Work out the finished part from the listing and answer in its coordinate system (mm). Face numbers are marked on the shaded views. A direction names the side the tool comes from. Round coordinates to 2 decimals unless told otherwise and drop trailing zeros. Write each loop counter-clockwise with the first axis right and the second up, starting at its lowest first coordinate (ties: lowest second). Pieces come first, ordered by that corner, then holes. Notation, with made-up numbers: (-15, -0.5) - (-4, -0.5) arc R26 cw to (-4, 22.5) - close; hole circle Ø7 at (-26.5, 66). An arc over 180 degrees is marked (long way). Write item = value, one per line. Start each with the question number.
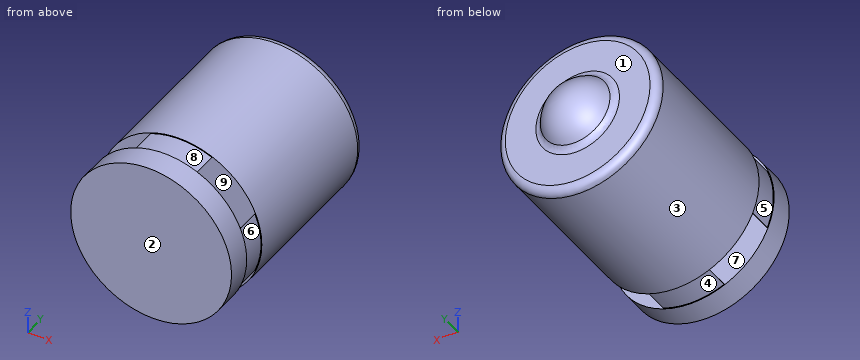
from build123d import *

# Parameters (mm, degrees)
SKETCH1_R           = 100
BOSS_EXTRUDE1_DEPTH = 30
BOSS_EXTRUDE2_DEPTH = 30
SKETCH3_R           = 100
BOSS_EXTRUDE3_DEPTH = 200
FILLET1_R           = 10
SCALE1_SCALE        = 0.233333333


with BuildPart() as part:
    # Sketch1 → Boss-Extrude1 (new body)
    with BuildSketch(Plane(origin=(0, 0, 0), x_dir=(1, 0, 0), z_dir=(0, 1, 0))):
        Circle(SKETCH1_R)
    extrude(amount=BOSS_EXTRUDE1_DEPTH)

    # Sketch2 → Boss-Extrude2 (add)
    with BuildSketch(Plane(origin=(0, 30, 0), x_dir=(1, 0, 0), z_dir=(0, 1, 0))):
        with BuildLine():
            Line((91.464073719, 37.885659804), (91.002133952, 37.694318088))
            ThreePointArc((91.002133952, 37.694318088), (98.5, 0), (91.002133952, -37.694318088))
            Line((91.002133952, -37.694318088), (91.464073719, -37.885659804))
            ThreePointArc((91.464073719, -37.885659804), (99, 0), (91.464073719, 37.885659804))
        make_face()
        with BuildLine():
            Line((37.885659804, -91.464073719), (37.694318088, -91.002133952))
            ThreePointArc((37.694318088, -91.002133952), (0, -98.5), (-37.694318088, -91.002133952))
            Line((-37.694318088, -91.002133952), (-37.885659804, -91.464073719))
            ThreePointArc((-37.885659804, -91.464073719), (0, -99), (37.885659804, -91.464073719))
        make_face()
        with BuildLine():
            Line((-91.464073719, -37.885659804), (-91.002133952, -37.694318088))
            ThreePointArc((-91.002133952, -37.694318088), (-98.5, 0), (-91.002133952, 37.694318088))
            Line((-91.002133952, 37.694318088), (-91.464073719, 37.885659804))
            ThreePointArc((-91.464073719, 37.885659804), (-99, 0), (-91.464073719, -37.885659804))
        make_face()
        with BuildLine():
            Line((-37.885659804, 91.464073719), (-37.694318088, 91.002133952))
            ThreePointArc((-37.694318088, 91.002133952), (0, 98.5), (37.694318088, 91.002133952))
            Line((37.694318088, 91.002133952), (37.885659804, 91.464073719))
            ThreePointArc((37.885659804, 91.464073719), (0, 99), (-37.885659804, 91.464073719))
        make_face()
    extrude(amount=BOSS_EXTRUDE2_DEPTH)

    # Sketch3 → Boss-Extrude3 (add)
    with BuildSketch(Plane(origin=(0, 60, 0), x_dir=(1, 0, 0), z_dir=(0, 1, 0))):
        Circle(SKETCH3_R)
    extrude(amount=BOSS_EXTRUDE3_DEPTH)

    # Sketch5 → Revolve1 (revolve)
    with BuildSketch(Plane.XY):
        with BuildLine():
            Line((45.82575695, 260), (0, 260))
            Line((0, 260), (0, 290))
            ThreePointArc((0, 290), (27.386127875, 281.833001327), (45.82575695, 260))
        make_face()
    revolve(axis=Axis((0, 115.728499237, 0), (0, 1, 0)))

    # Fillet1
    fillet1_edges = [part.edges().sort_by_distance(p)[0] for p in [
        (-100, 260, 0),
        (-45.82575695, 260, 0),
    ]]
    fillet(fillet1_edges, radius=FILLET1_R)


with BuildPart() as part_1:
    # Scale1: scaled about (-2.1e-08, 142.843087279, 0)
    add(part.part.scale(SCALE1_SCALE).moved(Location((-1.6e-08, 109.513033581, 0))))


solid = part_1.part
1. Each of these flat-tipped pins is pushed along its axis until it touches: pin 1 (12 mm diameter, centred on x = -18, y = 121.5, fed in from +Z); pin 2 (4 mm diameter, centred on x = -8.5, z = 5.5, fed in from +Y); pin 3 (3 mm diameter, centred on x = 18, y = 127, fed in from -Z). Where does it stop, or does it pass through?
2. Consider line 1 (Y direction, x = 17.5, z = -10.5); line 2 (Y direction, x = 5, z = -3); line 3 (Z direction, x = -2.5, y = 152). Determine where each line is inside the solid, lowest interval first.
3. Which of the six approach directions +Z, -Z, +X, -X, +Y, -Y give full straight-line access (tool end or side, diameter ignored) to the marked faces 1, 2, 3, 4 and 5?
4. For a pull along Z with two mould halves and no side action, classify the marked faces 6, 7, 8 and 9 as released by +Z, released by -Z, zero draft, split by the parting line, or undercut.
5. Find section A-A on y = 151. Give the vertices of the cut face in (x, z), plus the area to 3 significant figures.
Answer key:
q1.pin_1 = 19.8
q1.pin_2 = 173.89
q1.pin_3 = -16.5
q2.line_1 = 109.51 to 116.51, 123.51 to 170.18
q2.line_2 = 109.51 to 116.51, 123.51 to 175.62
q2.line_3 = -23.2 to 23.2
q3.face_1 = +Y
q3.face_2 = +Z, -Z, +X, -X, -Y
q3.face_3 = +Y, -Y
q3.face_4 = -Z
q3.face_5 = -X
q4.face_6 = split by the parting line
q4.face_7 = undercut
q4.face_8 = released by +Z
q4.face_9 = undercut
q5.outline = circle Ø46.67 at (0, 0)
q5.area = 1,710 mm²
